Verification items for the finished model (mm, model axes). A direction names the side the tool comes from. Coordinates: 2 decimals unless noted, no trailing zeros. Loops run counter-clockwise (first coordinate to the right, second up) from the corner with the lowest first, then second, coordinate; pieces in that order, holes last. Notation, with made-up numbers: (14.5, 63) - (73.5, 63) arc R6 ccw to (73.5, 73) - close; hole circle Ø2 at (27, 62.5). An arc over 180 degrees is marked (long way). One line per item, written item: value. Start each with the question number.
(1) Section check A-A (z = -9). Record the boundary of the cut face in (x, y).
(2) Gauge pin test, flat ends, axial feed: P1, Ø0.8, axis at x = -10.5, y = 2, coming from the +Z side; P2, Ø6, axis at x = -7.5, z = -7.5, coming from the +Y side. Record the tip position at first contact, or that the pin passes through.
(3) Section check C-C (x = -5.5). Record the boundary of the cut face in (y, z).
(4) Section check D-D (z = -38.5). Record the boundary of the cut face in (x, y).
(5) Draft check along X on faces 1 (the face through (-6.774, 18, -41)), 2 (the face through (-9.56, 10.17, -41.09)), 3 (the face through (-5, 20, -41)), 4 (the face through (-15.765, 4, -29)). Enter one of: +X half, -X half, draft (parallel to the pull), parting line (faces both ways), or undercut.
(6) Section check B-B (y = 15). Record the boundary of the cut face in (x, z), plus the area to 3 significant figures.
(7) Thickness scan on probe 1 along Y at (x, z) = (-8, -9); probe 2 along Y at (x, z) = (-12.25, -23.5); probe 3 along Z at (x, y) = (-6.75, 1.25). Record the ranges inside material, lowest first. Write a range as [from, to].
(8) Set-up check for faces 5 (the face through (-10, 3, -18.059)), 6 (the face through (-10, 8, -43.059)), 7 (the face through (-12.772, 18, -41)), 8 (the face through (-10, 9, -39.059)): record each of +Z, -Z, +X, -X, +Y, -Y from which the full face is reachable in a straight line by a thin tool's end or side.
```python
from build123d import *

# Parameters (mm, degrees)
SKETCH2_W           = 12
SKETCH2_H           = 40
BOSS_EXTRUDE1_DEPTH = 5
SKETCH3_W           = 12.004104261
SKETCH3_H           = 2.6
CUT_EXTRUDE1_DEPTH  = 15
SKETCH4_W           = 12
SKETCH4_H           = 4
BOSS_EXTRUDE2_DEPTH = 15
SKETCH5_R           = 3.75
CUT_EXTRUDE2_DEPTH  = 15
SKETCH6_W           = 5.997636367
SKETCH6_H           = 3.881980202
CUT_EXTRUDE3_DEPTH  = 10


with BuildPart() as part:
    # Sketch2 → Boss-Extrude1 (new body)
    with BuildSketch(Plane(origin=(0, 0, 0), x_dir=(1, 0, 0), z_dir=(0, 1, 0))):
        with Locations((-9.764705882, 23.058823529)):
            Rectangle(SKETCH2_W, SKETCH2_H)
    extrude(amount=BOSS_EXTRUDE1_DEPTH)

    # Sketch3 → Cut-Extrude1 (cut)
    with BuildSketch(Plane.XY.offset(-3.058823529)):
        with Locations((-9.766758013, 2.489565118)):
            Rectangle(SKETCH3_W, SKETCH3_H)
    extrude(amount=-CUT_EXTRUDE1_DEPTH, mode=Mode.SUBTRACT)

    # Sketch4 → Boss-Extrude2 (add)
    with BuildSketch(Plane(origin=(0, 5, 0), x_dir=(1, 0, 0), z_dir=(0, 1, 0))):
        with Locations((-9.764705882, 41.058823529)):
            Rectangle(SKETCH4_W, SKETCH4_H)
    extrude(amount=BOSS_EXTRUDE2_DEPTH)

    # Sketch5 → Cut-Extrude2 (cut)
    with BuildSketch(Plane(origin=(0, 0, -43.058823529), x_dir=(-1, 0, 0), z_dir=(0, 0, -1))):
        with Locations((9.734798195, 13.917907096)):
            Circle(SKETCH5_R)
    extrude(amount=-CUT_EXTRUDE2_DEPTH, mode=Mode.SUBTRACT)

    # Sketch6 → Cut-Extrude3 (cut)
    with BuildSketch(Plane(origin=(0, 0, -43.058823529), x_dir=(-1, 0, 0), z_dir=(0, 0, -1))):
        with Locations((9.772755291, 18.059009899)):
            Rectangle(SKETCH6_W, SKETCH6_H)
    extrude(amount=-CUT_EXTRUDE3_DEPTH, mode=Mode.SUBTRACT)


solid = part.part
```
Responses:
1. outline: (-15.76, 0) - (-3.76, 0) - (-3.76, 1.19) - (-15.76, 1.19) - close; (-15.76, 3.79) - (-3.76, 3.79) - (-3.76, 5) - (-15.76, 5) - close
2. P1: stops at z = -18.06
2. P2: stops at y = 5
3. outline: (0, -43.06) - (20, -43.06) - (20, -39.06) - (5, -39.06) - (5, -3.06) - (3.79, -3.06) - (3.79, -18.06) - (1.19, -18.06) - (1.19, -3.06) - (0, -3.06) - close
4. outline: (-15.76, 0) - (-3.76, 0) - (-3.76, 5) - (-15.76, 5) - close
5. face 1: undercut
5. face 2: undercut
5. face 3: draft
5. face 4: -X half
6. outline: (-15.76, -43.06) - (-13.33, -43.06) - (-13.33, -39.06) - (-15.76, -39.06) - close; (-6.14, -43.06) - (-3.76, -43.06) - (-3.76, -39.06) - (-6.14, -39.06) - close
6. area: 19.3 mm²
7. probe 1: y = [0, 1.19], [3.79, 5]
7. probe 2: y = [0, 5]
7. probe 3: z = [-43.06, -18.06]
8. face 5: +Z, +X, -X
8. face 6: -Z, +X, -X, +Y, -Y
8. face 7: +Z, -Z, +Y
8. face 8: +Z, +X, -X, +Y
